The model under review builds one solid part; all positions refer to its coordinate system, in mm. A direction names the side the tool comes from. Give positions to 0.01 mm unless a question says otherwise; leave off trailing zeros. Write each loop counter-clockwise with the first axis right and the second up, starting at its lowest first coordinate (ties: lowest second). Pieces come first, ordered by that corner, then holes. Notation, with made-up numbers: (16, 78) - (69, 78) arc R17 ccw to (69, 97) - close; hole circle Ø1 at (26.25, -7). An arc over 180 degrees is marked (long way). Write item = value, one per line.
```python
from build123d import *

# Parameters (mm, degrees)
F1_DEPTH = 1000


with BuildPart() as f1:
    # F0 (on Front) → F1 (new body)
    with BuildSketch(Plane.XZ):
        Polygon((0, 29.880688), (0, 0), (10.851949, 0), (10.851949, 22.142284), (33.172444, 22.142284), (33.172444, 29.880688), align=None)
        Polygon((0, 0), (-10.851949, 0), (-10.851949, -22.142284), (-33.172444, -22.142284), (-33.172444, -29.880688), (0, -29.880688), (33.172444, -29.880688), (33.172444, -22.142284), (10.851949, -22.142284), (10.851949, 0), align=None)
        Polygon((-10.851949, 22.142284), (-10.851949, 0), (0, 0), (0, 29.880688), (-33.172444, 29.880688), (-33.172444, 22.142284), align=None)
    extrude(amount=-F1_DEPTH)


solid = f1.part
```
1. Take a section at C-C on z = -4. Give the boundary of the cut face in (x, y).
Findings below:
outline = (-10.85, 0) - (10.85, 0) - (10.85, 1000) - (-10.85, 1000) - close
2. Draft analysis for pull direction Z (two halves, no side actions). For faces 1 (the flat face through (0, 493, 29.881)), 2 (the flat face through (-10.852, 493, 0)), 3 (the flat face through (0, 1000, 0)), state which applies: +Z half, -Z half, draft (parallel to the pull), parting line (faces both ways), or undercut.
Findings below:
face_1 = +Z half
face_2 = undercut
face_3 = draft
3. Take a section at B-B on y = 424. Give the boundary of the cut face in (x, z), and give its area (3 significant figures).
Findings below:
outline = (-33.17, -29.88) - (33.17, -29.88) - (33.17, -22.14) - (10.85, -22.14) - (10.85, 22.14) - (33.17, 22.14) - (33.17, 29.88) - (-33.17, 29.88) - (-33.17, 22.14) - (-10.85, 22.14) - (-10.85, -22.14) - (-33.17, -22.14) - close
area = 1,990 mm²
4. Machinability: for faces 4 (the flat face through (-22, 493, -22.142)), 5 (the flat face through (22, 493, -22.142)), 6 (the flat face through (0, 493, -29.881)), which of the approach directions +Z, -Z, +X, -X, +Y, -Y give a long, thin tool a straight path to every point of the face, cutting with its end or side? Answer none if there is none.
Findings below:
face_4 = -X, +Y, -Y
face_5 = +X, +Y, -Y
face_6 = -Z, +X, -X, +Y, -Y
5. Take a section at A-A on x = 23. Give the boundary of the cut face in (y, z), and give its area (3 significant figures).
Findings below:
outline = (0, -29.88) - (1000, -29.88) - (1000, -22.14) - (0, -22.14) - close; (0, 22.14) - (1000, 22.14) - (1000, 29.88) - (0, 29.88) - close
area = 15,500 mm²
6. For line 1 (Z direction, x = -24.5, y = 855); line 2 (X direction, y = 735, z = -8.5), list the stretches that pass through material, from the lowest coordinate up. Write a range as from..to.
Findings below:
line_1 = -29.88..-22.14, 22.14..29.88
line_2 = -10.85..10.85
7. Insertion check: P1, Ø13.5, axis at y = 274.5, z = 1.5, coming from the -X side. The pin has a flat end and moves straight along its axis. Give the tip position at first contact, or say it passes through.
Findings below:
P1 = -10.85
